Source: CAD feature listing. Evaluate the final solid. Frame: model axes, mm. Coordinates: 2 decimals unless noted, no trailing zeros. Loops run counter-clockwise (first coordinate to the right, second up) from the corner with the lowest first, then second, coordinate; pieces in that order, holes last.
Item 1: Line query: probe 1 along X at (y, z) = (81.28, 0.2); probe 2 along X at (y, z) = (81.5, 0.15); probe 3 along Y at (x, z) = (96.52, 0.35). Output: solid intervals per line, ascending.
Item 2: Section query C-C, the plane y = 76.75. Return the cut outline in (x, z).
Item 3: Section query B-B, the plane z = 0.25. Return the cut outline in (x, y), then the cut area to 3 significant figures.
Item 4: Section query A-A, the plane x = 101.6. Return the cut outline in (y, z).
Item 5: Section query D-D, the plane x = 96.52. Return the cut outline in (y, z).
Item 6: Pull-direction query (Y, two-part tool) for faces 1 (the flat face through (97, 74, 0)), 2 (the cylindrical face through (97.79, 75.87, 0.2)); classes: +Y half, -Y half, draft (parallel to the pull), parting line (faces both ways), or undercut.
```python
from build123d import *

# Parameters (mm, degrees)
SKETCH1_W           = 15.748
SKETCH1_H           = 19.812
SKETCH1_R           = 1.27
SKETCH1_R_2         = 0.952
SKETCH1_R_3         = 0.381
BOSS_EXTRUDE1_DEPTH = 0.41148


with BuildPart() as part:
    # Sketch1 → Boss-Extrude1 (new body)
    with BuildSketch(Plane(origin=(0, 0, 0), x_dir=(-1, 0, 0), z_dir=(0, 0, -1))):
        with Locations((-96.52, 73.914)):
            Rectangle(SKETCH1_W, SKETCH1_H)
        with Locations((-96.52, 75.819)):
            Circle(SKETCH1_R, mode=Mode.SUBTRACT)
        with Locations((-91.44, 81.28)):
            Circle(SKETCH1_R_2, mode=Mode.SUBTRACT)
        with Locations(Location((-96.52, 68.453, 0), (0, 0, 180))):
            Circle(SKETCH1_R_3, mode=Mode.SUBTRACT)
        with Locations((-101.6, 81.28)):
            Circle(SKETCH1_R_2, mode=Mode.SUBTRACT)
    extrude(amount=-BOSS_EXTRUDE1_DEPTH)


solid = part.part
```
Verdict:
1. probe 1: x = 88.65 to 90.49, 92.39 to 100.65, 102.55 to 104.39
1. probe 2: x = 88.65 to 90.51, 92.37 to 100.67, 102.53 to 104.39
1. probe 3: y = 64.01 to 68.07, 68.83 to 74.55, 77.09 to 83.82
2. outline: (88.65, 0) - (95.66, 0) - (95.66, 0.41) - (88.65, 0.41) - close; (97.38, 0) - (104.39, 0) - (104.39, 0.41) - (97.38, 0.41) - close
3. outline: (88.65, 64.01) - (104.39, 64.01) - (104.39, 83.82) - (88.65, 83.82) - close; hole circle Ø1.9 at (91.44, 81.28); hole circle Ø2.54 at (96.52, 75.82); hole circle Ø0.76 at (96.52, 68.45); hole circle Ø1.9 at (101.6, 81.28)
3. area: 301 mm2
4. outline: (64.01, 0) - (80.33, 0) - (80.33, 0.41) - (64.01, 0.41) - close; (82.23, 0) - (83.82, 0) - (83.82, 0.41) - (82.23, 0.41) - close
5. outline: (64.01, 0) - (68.07, 0) - (68.07, 0.41) - (64.01, 0.41) - close; (68.83, 0) - (74.55, 0) - (74.55, 0.41) - (68.83, 0.41) - close; (77.09, 0) - (83.82, 0) - (83.82, 0.41) - (77.09, 0.41) - close
6. face 1: draft
6. face 2: undercut
